from build123d import *

# Parameters (mm, degrees)
SKETCH8_R          = 50.8
CUT_EXTRUDE3_DEPTH = 50.8


with BuildPart() as part:
    # Sketch1 → Revolve2 (revolve)
    with BuildSketch(Plane.XY, mode=Mode.PRIVATE) as revolve2_sk:
        Polygon((0, 101.6), (101.6, 101.6), (101.6, 0), (0, 0), (-25.4, 0), (-127, 0), (-127, 101.6), (-25.4, 101.6), (-25.4, 82.55), (0, 82.55), align=None)
    revolve(revolve2_sk.sketch.rotate(Axis((141.005607477, 0, 0), (-1, 0, 0)), 90), axis=Axis((141.005607477, 0, 0), (-1, 0, 0)))

    # Sketch8 → Cut-Extrude3 (cut)
    with BuildSketch(Plane(origin=(101.6, 0, 0), x_dir=(0, 0, -1), z_dir=(1, 0, 0))):
        Circle(SKETCH8_R)
    extrude(amount=-CUT_EXTRUDE3_DEPTH, mode=Mode.SUBTRACT)

    # Cut-Loft1: read off the stored shape, not the designer's step
    # Cut-Loft1: loft between two sections, ruled curve by curve
    cut_loft1_from = [
        Edge.make_bspline([(-127, 1.659470947, -50.772888003), (-127, 103.205246954, -47.453946108), (-127, 99.886305059, 54.091829898), (-127, -1.659470947, 50.772888003), (-127, -103.205246954, 47.453946108), (-127, -99.886305059, -54.091829898), (-127, 1.659470947, -50.772888003)], [0, 0, 0, 0, 0.5, 0.5, 0.5, 1, 1, 1, 1], 3, [1, 0.333333333, 0.333333333, 1, 0.333333333, 0.333333333, 1]),
    ]
    cut_loft1_to = [
        Edge.make_bspline([(-57.15, -3.878953486, -12.093126967), (-57.15, 20.307300449, -19.85103394), (-57.15, 28.065207421, 4.335219995), (-57.15, 3.878953486, 12.093126967), (-57.15, -20.307300449, 19.85103394), (-57.15, -28.065207421, -4.335219995), (-57.15, -3.878953486, -12.093126967)], [0, 0, 0, 0, 0.5, 0.5, 0.5, 1, 1, 1, 1], 3, [1, 0.333333333, 0.333333333, 1, 0.333333333, 0.333333333, 1]),
    ]
    cut_loft1 = Solid(Shell([*[Face.make_surface_from_curves(cut_loft1_from[k], cut_loft1_to[k]) for k in range(1)], Face(Wire(cut_loft1_from)), Face(Wire(cut_loft1_to))]))
    add(cut_loft1, mode=Mode.SUBTRACT)


solid = part.part
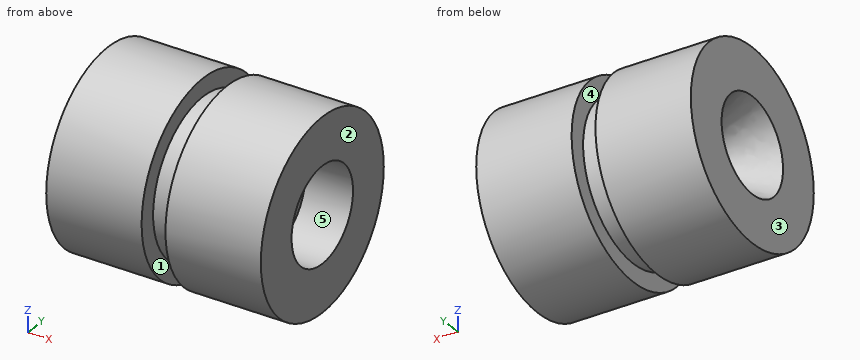
Check sheet for the modelled part. Datum: model origin and axes. Units: mm. Face numbers are marked on the shaded views. A direction names the side the tool comes from. Round coordinates to 2 decimals unless told otherwise and drop trailing zeros. Loops run counter-clockwise (first coordinate to the right, second up) from the corner with the lowest first, then second, coordinate; pieces in that order, holes last.
1. Gauge pin test, flat ends, axial feed: pin 1 Ø10 at (y, z) = (33.5, 4.5) entering from +X; pin 2 Ø1 at (x, y) = (-62.5, 54.5) entering from +Z; pin 3 Ø8 at (x, z) = (11.5, -53.5) entering from -Y. Record the tip position at first contact, or that the pin passes through.
2. Mould release check, pull along X, two halves, no side actions. Record for the marked faces 3, 4 and 5: released by +X, released by -X, zero draft, split by the parting line, or undercut.
3. Set-up check for the marked faces 1 and 2: record each of +Z, -Z, +X, -X, +Y, -Y from which the full face is reachable in a straight line by a thin tool's end or side.
4. Sectioned sample at B-B on z = -58.5. Record the boundary of the cut face in (x, y).
5. Scan lines: probe 1 along X at (y, z) = (-72, -48); probe 2 along Y at (x, z) = (72, 0); probe 3 along Z at (x, y) = (67, 28.5). Record each from-to range of solid material in increasing order.
6. Sectioned sample at A-A on x = 71. Record the boundary of the cut face in (y, z).
7. Sectioned sample at C-C on x = -45.5. Record the boundary of the cut face in (y, z).
8. Sectioned sample at D-D on z = 67. Record the boundary of the cut face in (x, y), and give its area (3 significant figures).
Recorded:
1. pin 1: stops at x = 50.8
1. pin 2: stops at z = 86.06
1. pin 3: stops at y = -88.73
2. face 3: released by -X
2. face 4: undercut
2. face 5: zero draft
3. face 1: none
3. face 2: +Z, -Z, +X, +Y, -Y
4. outline: (-127, -83.07) - (-25.4, -83.07) - (-25.4, -58.24) - (0, -58.24) - (0, -83.07) - (101.6, -83.07) - (101.6, 83.07) - (0, 83.07) - (0, 58.24) - (-25.4, 58.24) - (-25.4, 83.07) - (-127, 83.07) - close
5. probe 1: x = -127 to -25.4, 0 to 101.6
5. probe 2: y = -101.6 to -50.8, 50.8 to 101.6
5. probe 3: z = -97.52 to -42.05, 42.05 to 97.52
6. outline: circle Ø203.2 at (0, 0); hole circle Ø101.6 at (0, 0)
7. outline: circle Ø203.2 at (0, 0)
8. outline: (-127, -76.38) - (-25.4, -76.38) - (-25.4, -48.22) - (0, -48.22) - (0, -76.38) - (101.6, -76.38) - (101.6, 76.38) - (0, 76.38) - (0, 48.22) - (-25.4, 48.22) - (-25.4, 76.38) - (-127, 76.38) - close
8. area: 33,500 mm2
